```python
from build123d import *

# Parameters (mm, degrees)
SKETCH1_R           = 127
BOSS_EXTRUDE1_DEPTH = 1016


with BuildPart() as part:
    # Sketch1 → Boss-Extrude1 (new body)
    with BuildSketch(Plane.XY):
        Circle(SKETCH1_R)
    extrude(amount=BOSS_EXTRUDE1_DEPTH)

    # Sketch6 → 3/8 Rc Tapped Hole2 (revolve, cut)
    with BuildSketch(Plane(origin=(0, 2.353512808, 1016), x_dir=(0, -1, 0), z_dir=(1, 0, 0))):
        Polygon((0, 0), (0, 1016), (25, 1016), (25, 20.32), (7.985917585, 20.32), (8.6094525, 0.3455475), (8.955, 0), align=None)
    revolve(axis=Axis((0, 2.353512808, 1022.35), (0, 0, -1)), mode=Mode.SUBTRACT)


solid = part.part
```
Could you check a few things on this model? Use its own coordinates, in mm. A direction names the side the tool comes from. Coordinates: 2 decimals unless noted, no trailing zeros. Order: outer loops, then holes, each group sorted by start corner. A loop starts at its lowest first (then second) coordinate and runs counter-clockwise, first axis right, second up. Notation, with made-up numbers: M 58,-31.75 L 70,-31.75 A24 cw 70,7.25 Z; hole C 70,43.5 d6. An arc over 180 degrees is marked long. Use one line per item in the form item = value. Start each with the question number.
1. Please list where these lines run through material, in increasing order: line 1 (Y direction, x = 0, z = 401); line 2 (X direction, y = -12, z = 784.5); line 3 (X direction, y = -19.5, z = 933).
2. Suppose I cut it at A-A on z = 404.5. Write out the boundary of the cut face in (x, y), then the cut area to 3 significant figures.
3. For pin 1 (3 mm diameter, centred on y = -39, z = 836, fed in from -X); pin 2 (8 mm diameter, centred on y = -98, z = 752, fed in from +X); pin 3 (10 mm diameter, centred on y = 86.5, z = 544.5, fed in from +X), each with a flat end and sliding along its axis, tell me the tip position at first contact or that it passes through.
4. Suppose I cut it at B-B on x = -69. Write out the boundary of the cut face in (y, z), then the cut area to 3 significant figures.
5. We'd pull the mould along X, two halves only. Please class faces 1 (the conical face through (5.052, 8.942, 1005.807)), 2 (the flat face through (26, 2, 1016)), 3 (the cylindrical face through (-27.53, -123.98, 500.89)): +X half, -X half, draft (parallel to the pull), parting line (faces both ways), or undercut.
6. Suppose I cut it at C-C on y = -82. Write out the boundary of the cut face in (x, z), then the cut area to 3 significant figures.
7. On a 3-axis mill with a long thin cutter (end or side, diameter ignored), from which of +Z, -Z, +X, -X, +Y, -Y can I reach the whole of each face in a straight line? I mean faces 4 (the flat face through (-6, 8, 995.68)), 5 (the flat face through (26, 2, 0)). Say none if no direction works.
Geometry says:
q1.line_1 = -127 to -22.65, 27.35 to 127
q1.line_2 = -126.43 to -20.47, 20.47 to 126.43
q1.line_3 = -125.49 to -12.14, 12.14 to 125.49
q2.outline = C 0,0 d254; hole C 0,2.35 d50
q2.area = 48,700 mm^2
q3.pin_1 = -121.34
q3.pin_2 = 85.4
q3.pin_3 = 97.4
q4.outline = M -106.62,0 L 106.62,0 L 106.62,1016 L -106.62,1016 Z
q4.area = 217,000 mm^2
q5.face_1 = undercut
q5.face_2 = draft
q5.face_3 = parting line
q6.outline = M -96.98,0 L 96.98,0 L 96.98,1016 L -96.98,1016 Z
q6.area = 197,000 mm^2
q7.face_4 = -Z
q7.face_5 = -Z, +X, -X, +Y, -Y
